```python
from build123d import *

# Parameters (mm, degrees)
F1_DEPTH = 7
F2_W     = 20
F2_H     = 10
F3_DEPTH = 7.001
F5_DEPTH = 7.001
F7_DEPTH = 7.001
F9_D     = 3.3
F11_D    = 3.3
F13_D    = 3.3


with BuildPart() as f1:
    # F0 (on Front) → F1 (new body)
    with BuildSketch(Plane.XZ):
        with BuildLine():
            ThreePointArc((-7.3612159322, -4.25), (-7.3612159322, 4.25), (0, 8.5))
            Line((0, 8.5), (0, 16))
            ThreePointArc((0, 16), (-13.8564064606, 8), (-13.8564064606, -8))
            Line((-13.8564064606, -8), (-7.3612159322, -4.25))
        make_face()
        Polygon((-20, 16), (0, 16), (20, 16), (20, 24), (-20, 24), align=None)
        with BuildLine():
            ThreePointArc((-13.8564064606, -8), (-13.8564064606, 8), (0, 16))
            Line((0, 16), (-20, 16))
            Line((-20, 16), (-23.8564064606, 9.3205080757))
            Line((-23.8564064606, 9.3205080757), (-13.8564064606, -8))
        make_face()
        Polygon((-3.8564064606, -25.3205080757), (-13.8564064606, -8), (-23.8564064606, 9.3205080757), (-30.7846096908, 5.3205080757), (-10.7846096908, -29.3205080757), align=None)
        with BuildLine():
            Line((13.8564064606, -8), (7.3612159322, -4.25))
            ThreePointArc((7.3612159322, -4.25), (0, -8.5), (-7.3612159322, -4.25))
            Line((-7.3612159322, -4.25), (-13.8564064606, -8))
            ThreePointArc((-13.8564064606, -8), (0, -16), (13.8564064606, -8))
        make_face()
        with BuildLine():
            Line((3.8564064606, -25.3205080757), (13.8564064606, -8))
            ThreePointArc((13.8564064606, -8), (0, -16), (-13.8564064606, -8))
            Line((-13.8564064606, -8), (-3.8564064606, -25.3205080757))
            Line((-3.8564064606, -25.3205080757), (3.8564064606, -25.3205080757))
        make_face()
        Polygon((23.8564064606, 9.3205080757), (13.8564064606, -8), (3.8564064606, -25.3205080757), (10.7846096908, -29.3205080757), (30.7846096908, 5.3205080757), align=None)
        with BuildLine():
            ThreePointArc((0, 8.5), (6.0104076401, 6.0104076401), (8.5, 0))
            ThreePointArc((8.5, 0), (8.2103695235, -2.1999618834), (7.3612159322, -4.25))
            Line((7.3612159322, -4.25), (13.8564064606, -8))
            ThreePointArc((13.8564064606, -8), (15.4548132206, -4.1411047216), (16, 0))
            ThreePointArc((16, 0), (11.313708499, 11.313708499), (0, 16))
            Line((0, 16), (0, 8.5))
        make_face()
        with BuildLine():
            Line((20, 16), (0, 16))
            ThreePointArc((0, 16), (11.313708499, 11.313708499), (16, 0))
            ThreePointArc((16, 0), (15.4548132206, -4.1411047216), (13.8564064606, -8))
            Line((13.8564064606, -8), (23.8564064606, 9.3205080757))
            Line((23.8564064606, 9.3205080757), (20, 16))
        make_face()
    extrude(amount=F1_DEPTH)

    # F2 (on face) → F3 (cut, through all)
    with BuildSketch(Plane.XZ.offset(7)):
        with Locations((0, 19)):
            Rectangle(F2_W, F2_H)
    extrude(amount=-F3_DEPTH, mode=Mode.SUBTRACT)

    # F4 (on face) → F5 (cut, through all)
    with BuildSketch(Plane.XZ.offset(7)):
        Polygon((7.124355653, -15.6602540378), (15.7846096908, -20.6602540378), (25.7846096908, -3.3397459622), (17.124355653, 1.6602540378), align=None)
    extrude(amount=-F5_DEPTH, mode=Mode.SUBTRACT)

    # F6 (on face) → F7 (cut, through all)
    with BuildSketch(Plane.XZ.offset(7)):
        Polygon((-15.7846096908, -20.6602540378), (-7.124355653, -15.6602540378), (-17.124355653, 1.6602540378), (-25.7846096908, -3.3397459622), align=None)
    extrude(amount=-F7_DEPTH, mode=Mode.SUBTRACT)

    # F9 (through all)
    with Locations(Plane(origin=(-20, 0, 0), x_dir=(0, -1, 0), z_dir=(-1, 0, 0))):
        with Locations((3.5, 20)):
            Hole(F9_D / 2)

    # F11 (through all)
    with Locations(Plane(origin=(10, 0, 17.3205080757), x_dir=(0.8660254038, 0, -0.5), z_dir=(0.5, 0, 0.8660254038))):
        with Locations((20, -3.5)):
            Hole(F11_D / 2)

    # F13 (through all)
    with Locations(Plane(origin=(10, 0, -17.3205080757), x_dir=(0.8660254038, 0, 0.5), z_dir=(0.5, 0, -0.8660254038))):
        with Locations((-20, 3.5)):
            Hole(F13_D / 2)


solid = f1.part
```
Part model, mm, in its own coordinate system. A direction names the side the tool comes from. Round coordinates to 2 decimals unless told otherwise and drop trailing zeros. Write each loop counter-clockwise with the first axis right and the second up, starting at its lowest first coordinate (ties: lowest second). Pieces come first, ordered by that corner, then holes. Notation, with made-up numbers: M 0.5,67.5 L 5.5,67.5 A33 cw 5.5,96.5 Z; hole C 44,46 d1. An arc over 180 degrees is marked long. Answer as CSV lines item,"result". Start each with the question number.
1) Band-saw the part on C-C (x = 5). List the corners of the cut face in (y, z), then the cut area to 3 significant figures.
2) Drop flat-ended pins along their axis: pin 1 (3.5 mm diameter, centred on x = -1, y = -4, fed in from -Z); pin 2 (3.5 mm diameter, centred on y = -3.5, z = 21, fed in from -X); pin 3 (3 mm diameter, centred on x = -1, y = -5.5, fed in from +Z); pin 4 (2 mm diameter, centred on y = -3.5, z = 20, fed in from -X). Give the stop position or say it passes through.
3) Band-saw the part on A-A (z = 20). List the corners of the cut face in (x, y), then the cut area to 3 significant figures.
4) Band-saw the part on B-B (y = -1). List the corners of the cut face in (x, z).
5) Drill centre lines: L1, parallel to X at y = -0.75, z = 21; L2, parallel to X at y = -1.75, z = 0.5; L3, parallel to X at y = -5.5, z = -3. Where is each one in solid material? Low to high.
6) Which spindle directions (+Z, -Z, +X, -X, +Y, -Y) get a long thin tool onto all of the face, cutting with end or side? Do faces 5 (the face through (20.553, -3.549, -0.319)), 6 (the face through (12.194, -3.549, -6.879)), 7 (the face through (0, -4, 14)), 8 (the face through (-20, -3, 18)). Say none if no direction does.
7) Mould opens along Z. For faces 1 (the face through (-11.218, -3.996, -23.717)), 2 (the face through (15, -3, 24)), 3 (the face through (-13.32, -3.45, -24.93)), 4 (the face through (-10, -4, 18)) say: +Z half, -Z half, draft (parallel to the pull), parting line (faces both ways), or undercut.
8) Band-saw the part on D-D (x = -13). Count the separate pieces of the cut face and the enclosed holes in it, then the cut area to 3 significant figures.
Worked out:
1,outline,"M -7,-25.98 L 0,-25.98 L 0,-6.87 L -7,-6.87 Z; M -7,6.87 L 0,6.87 L 0,14 L -7,14 Z"
1,area,"184 mm²"
2,pin 1,"z = -25.32"
2,pin 2,"x = -20"
2,pin 3,"z = 14"
2,pin 4,"through"
3,outline,"M -20,-7 L -10,-7 L -10,-5.15 L -20,-5.15 Z; M -20,-1.85 L -10,-1.85 L -10,0 L -20,0 Z; M 10,-7 L 20,-7 L 20,-5.15 L 10,-5.15 Z; M 10,-1.85 L 20,-1.85 L 20,0 L 10,0 Z"
3,area,"74.0 mm²"
4,outline,"M -30.78,5.32 L -25.78,-3.34 L -17.12,1.66 L -7.12,-15.66 L -15.78,-20.66 L -10.78,-29.32 L -3.86,-25.32 L 3.86,-25.32 L 10.78,-29.32 L 15.78,-20.66 L 7.12,-15.66 L 17.12,1.66 L 25.78,-3.34 L 30.78,5.32 L 23.86,9.32 L 20,16 L 20,24 L 10,24 L 10,14 L -10,14 L -10,24 L -20,24 L -20,16 L -23.86,9.32 Z; hole C 0,0 d17"
5,L1,"-20 to -10, 10 to 20"
5,L2,"-28 to -19.13, -16.45 to -8.49, 8.49 to 16.45, 19.13 to 28"
5,L3,"-25.98 to -25.2, -14.43 to -7.95, 7.95 to 14.43, 25.2 to 25.98"
6,face 5,"-Z, +Y, -Y"
6,face 6,"+Y, -Y"
6,face 7,"+Z, +Y, -Y"
6,face 8,"+Z, -X, +Y, -Y"
7,face 1,"undercut"
7,face 2,"+Z half"
7,face 3,"-Z half"
7,face 4,"draft"
8,separate pieces,"2"
8,enclosed holes,"1"
8,area,"239 mm²"
